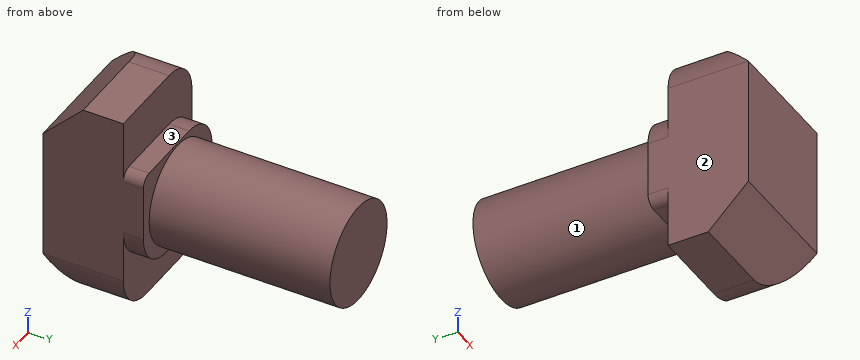
```python
from build123d import *

# Parameters (mm, degrees)
BOSS_EXTRUDE1_DEPTH = 3
FILLET1_R           = 2
FILLET2_R           = 2
FILLET3_R           = 0.5
SKETCH2_W           = 2.5
SKETCH2_H           = 9


with BuildPart() as part:
    # Sketch1 → Boss-Extrude1 (new body, symmetric)
    with BuildSketch(Plane(origin=(0, 0, 0), x_dir=(0, 0, -1), z_dir=(1, 0, 0))):
        Polygon((-2.625, 0), (2.625, 0), (2.625, -1), (5.25, -1), (5.25, -3), (3.25, -5), (-3.25, -5), (-5.25, -3), (-5.25, -1), (-2.625, -1), align=None)
    extrude(amount=BOSS_EXTRUDE1_DEPTH, both=True)

    # Fillet1
    fillet1_edges = [part.edges().sort_by_distance(p)[0] for p in [
        (3, -2, -5.25),
        (-3, -2, 5.25),
    ]]
    fillet(fillet1_edges, radius=FILLET1_R)

    # Fillet2
    fillet2_edges = [part.edges().sort_by_distance(p)[0] for p in [
        (-3, -0.5, 2.625),
        (3, -0.5, -2.625),
    ]]
    fillet(fillet2_edges, radius=FILLET2_R)

    # Fillet3
    fillet3_edges = [part.edges().sort_by_distance(p)[0] for p in [
        (3, -0.5, 2.625),
        (-3, -0.5, -2.625),
    ]]
    fillet(fillet3_edges, radius=FILLET3_R)

    # Sketch2 → Revolve1 (revolve)
    with BuildSketch(Plane.XY):
        with Locations((1.25, 4.5)):
            Rectangle(SKETCH2_W, SKETCH2_H)
    revolve(axis=Axis((0, 55, 0), (0, -1, 0)))


solid = part.part
```
Input: part model. Units: mm. Frame: model coordinates. Face numbers are marked on the shaded views. A direction names the side the tool comes from. Round coordinates to 2 decimals unless told otherwise and drop trailing zeros. Loops run counter-clockwise (first coordinate to the right, second up) from the corner with the lowest first, then second, coordinate; pieces in that order, holes last. Notation, with made-up numbers: (-19.5, 85) - (17.5, 85) arc R25 ccw to (17.5, 105) - close; hole circle Ø1 at (7, -12). An arc over 180 degrees is marked (long way). One line per item, written item: value. Start each with the question number.
(1) Ray query, line 1 (Y direction, x = -2.25, z = 2.5); line 2 (Y direction, x = 2.25, z = 1.5); line 3 (X direction, y = 3, z = 2.25). Return the intervals inside material, ascending. Write a range as [from, to].
(2) Section D-D, the plane z = -3. Return loops of the section in (x, y).
(3) Section A-A, the plane x = 0. Return loops of the section in (y, z) (3 decimals), plus the area to 4 significant figures.
(4) Contact query for flat-ended pins moving along their axis: P1, Ø0.8, axis at x = 0.5, y = -0.5, coming from the +Z side (3 decimals); P2, Ø0.5, axis at x = -0.5, y = -0.5, coming from the -Z side (3 decimals); P3, Ø1.5, axis at x = -1.5, y = 5, coming from the +Z side. Output: stop coordinate, or through.
(5) Section C-C, the plane y = 0.25. Return loops of the section in (x, z), plus the area to 3 significant figures.
(6) Access query for the marked faces 1, 2 and 3. Directions: +Z, -Z, +X, -X, +Y, -Y. A direction counts if a zero-diameter tool reaches every point of the face in a straight line with its end or side. Return the directions, or none.
(7) Section B-B, the plane z = 0. Return loops of the section in (x, y), plus the area to 3 significant figures.
Results below:
1. line 1: [-5, -1]
1. line 2: [-5, 0]
1. line 3: [-1.09, 1.09]
2. outline: (-3, -5) - (3, -5) - (3, -1) - (-3, -1) - close
3. outline: (-5, -3.25) - (-3, -5.25) - (-1, -5.25) - (-1, -2.625) - (0, -2.625) - (0, -2.5) - (9, -2.5) - (9, 2.5) - (0, 2.5) - (0, 2.625) - (-1, 2.625) - (-1, 5.25) - (-3, 5.25) - (-5, 3.25) - close
3. area: 88.25 mm^2
4. P1: z = 2.625
4. P2: z = -2.625
4. P3: z = 2.38
5. outline: circle Ø5 at (0, 0)
5. area: 19.6 mm^2
6. face 1: +Y
6. face 2: +Z, -Z, -X, +Y, -Y
6. face 3: +Z, +X, -X, +Y
7. outline: (-3, -5) - (3, -5) - (3, 0) - (2.5, 0) - (2.5, 9) - (-2.5, 9) - (-2.5, 0) - (-3, 0) - close
7. area: 75.0 mm^2
